The listing builds one solid part. Answer for the finished solid, in the listing's coordinates (mm). Give positions to 0.01 mm unless a question says otherwise; leave off trailing zeros. Write each loop counter-clockwise with the first axis right and the second up, starting at its lowest first coordinate (ties: lowest second). Pieces come first, ordered by that corner, then holes. Notation, with made-up numbers: M 45,25.25 L 70,25.25 A22 cw 70,36.25 Z; hole C 18,7 d7. An arc over 180 degrees is marked long. Return JSON: item names as keys, results as strings.
from build123d import *

# Parameters (mm, degrees)
SKETCH1_W           = 171.45
SKETCH1_H           = 127
BOSS_EXTRUDE1_DEPTH = 2.54
SKETCH2_W           = 2.54
SKETCH2_H           = 25.4
CUT_EXTRUDE1_DEPTH  = 3.54
SKETCH3_R           = 11.43
CUT_EXTRUDE2_DEPTH  = 3.54
SKETCH4_W           = 21.166666667
SKETCH4_H           = 2.54
CUT_EXTRUDE3_DEPTH  = 3.54


with BuildPart() as part:
    # Sketch1 → Boss-Extrude1 (new body)
    with BuildSketch(Plane(origin=(0, 0, 0), x_dir=(0, 0, -1), z_dir=(1, 0, 0))):
        with Locations((85.725, 63.5)):
            Rectangle(SKETCH1_W, SKETCH1_H)
    extrude(amount=BOSS_EXTRUDE1_DEPTH)

    # Sketch2 → Cut-Extrude1 (cut, through all)
    with BuildSketch(Plane(origin=(2.54, 0, 0), x_dir=(0, 0, -1), z_dir=(1, 0, 0))):
        with Locations((1.27, 88.9)):
            Rectangle(SKETCH2_W, SKETCH2_H)
        with Locations((1.27, 38.1)):
            Rectangle(SKETCH2_W, SKETCH2_H)
        with Locations((170.18, 88.9)):
            Rectangle(SKETCH2_W, SKETCH2_H)
        with Locations((170.18, 38.1)):
            Rectangle(SKETCH2_W, SKETCH2_H)
    extrude(amount=-CUT_EXTRUDE1_DEPTH, mode=Mode.SUBTRACT)

    # Sketch3 → Cut-Extrude2 (cut, through all)
    with BuildSketch(Plane(origin=(2.54, 0, 0), x_dir=(0, 0, -1), z_dir=(1, 0, 0))):
        with Locations((61.976, 63.5)):
            Circle(SKETCH3_R)
    extrude(amount=-CUT_EXTRUDE2_DEPTH, mode=Mode.SUBTRACT)

    # Sketch4 → Cut-Extrude3 (cut, through all)
    with BuildSketch(Plane(origin=(2.54, 0, 0), x_dir=(0, 0, -1), z_dir=(1, 0, 0))):
        with Locations((133.265333333, 1.27)):
            Rectangle(SKETCH4_W, SKETCH4_H)
    extrude(amount=-CUT_EXTRUDE3_DEPTH, mode=Mode.SUBTRACT)


solid = part.part
Item 1: A cutting plane is placed at B-B, the plane y = 63.5. Write down the section's boundary in (x, z).
Geometry results:
{"outline": "M 0,-171.45 L 2.54,-171.45 L 2.54,-73.41 L 0,-73.41 Z; M 0,-50.55 L 2.54,-50.55 L 2.54,0 L 0,0 Z"}
Item 2: Given pin 1 Ø1.3 at (x, y) = (0.5, 42.5) entering from +Z; pin 2 Ø1.3 at (x, y) = (1.5, 37) entering from -Z, each flat-ended and moving along its own axis, determine where each tip first touches the part or whether it passes through.
Geometry results:
{"pin 1": "stops at z = -2.54", "pin 2": "stops at z = -168.91"}
Item 3: A cutting plane is placed at C-C, the plane z = -58.5. Write down the section's boundary in (x, y).
Geometry results:
{"outline": "M 0,0 L 2.54,0 L 2.54,52.61 L 0,52.61 Z; M 0,74.39 L 2.54,74.39 L 2.54,127 L 0,127 Z"}
Item 4: A cutting plane is placed at D-D, the plane y = 98. Write down the section's boundary in (x, z), plus the area to 3 significant figures.
Geometry results:
{"outline": "M 0,-168.91 L 2.54,-168.91 L 2.54,-2.54 L 0,-2.54 Z", "area": "423 mm2"}
Item 5: Find the intervals of material crossed by line 1 (Z direction, x = 1.9, y = 68); line 2 (Y direction, x = 0.85, z = -142.5); line 3 (Y direction, x = 0.7, z = -66.5), in increasing order.
Geometry results:
{"line 1": "z = -171.45 to -72.48, -51.47 to 0", "line 2": "y = 2.54 to 127", "line 3": "y = 0 to 53, 74 to 127"}
Item 6: A cutting plane is placed at A-A, the plane x = 1.05. Write down the section's boundary in (y, z).
Geometry results:
{"outline": "M 0,-171.45 L 25.4,-171.45 L 25.4,-168.91 L 50.8,-168.91 L 50.8,-171.45 L 76.2,-171.45 L 76.2,-168.91 L 101.6,-168.91 L 101.6,-171.45 L 127,-171.45 L 127,0 L 101.6,0 L 101.6,-2.54 L 76.2,-2.54 L 76.2,0 L 50.8,0 L 50.8,-2.54 L 25.4,-2.54 L 25.4,0 L 0,0 L 0,-122.68 L 2.54,-122.68 L 2.54,-143.85 L 0,-143.85 Z; hole C 63.5,-61.98 d22.86"}
